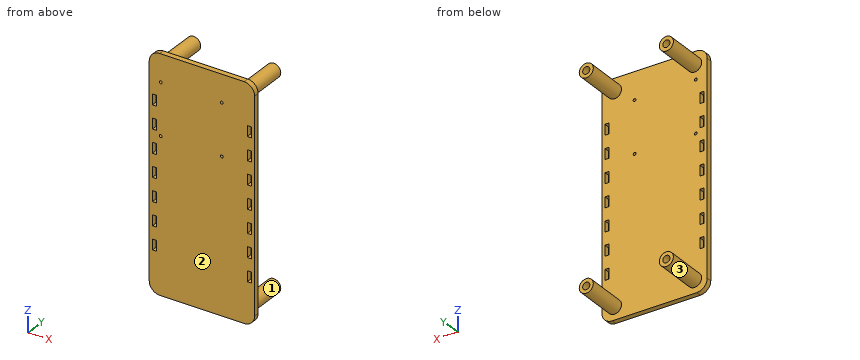
from build123d import *

# Parameters (mm, degrees)
SKETCH1_W           = 100
SKETCH1_H           = 220
BOSS_EXTRUDE1_DEPTH = 5
FILLET1_R           = 10
FILLET2_R           = 10
FILLET3_R           = 10
FILLET4_R           = 10
SKETCH2_R           = 6.668119003
BOSS_EXTRUDE2_DEPTH = 40
SKETCH4_R           = 3.418119003
CUT_EXTRUDE1_DEPTH  = 15
SKETCH5_R           = 3.418119003
CUT_EXTRUDE2_DEPTH  = 15
SKETCH6_R           = 3.418119003
CUT_EXTRUDE3_DEPTH  = 15
SKETCH7_R           = 3.418119003
CUT_EXTRUDE4_DEPTH  = 15
SKETCH8_W           = 4
SKETCH8_H           = 10
CUT_EXTRUDE5_DEPTH  = 157.908412776
SKETCH9_R           = 1.35
CUT_EXTRUDE7_DEPTH  = 159.256911381


with BuildPart() as part:
    # Sketch1 → Boss-Extrude1 (new body)
    with BuildSketch(Plane(origin=(0, 0, 0), x_dir=(1, 0, 0), z_dir=(0, 1, 0))):
        with Locations((-54.5, 0)):
            Rectangle(SKETCH1_W, SKETCH1_H)
    extrude(amount=BOSS_EXTRUDE1_DEPTH)

    # Fillet1
    fillet1_edges = [part.edges().sort_by_distance(p)[0] for p in [
        (-4.5, 2.5, 110),
    ]]
    fillet(fillet1_edges, radius=FILLET1_R)

    # Fillet2
    fillet2_edges = [part.edges().sort_by_distance(p)[0] for p in [
        (-4.5, 2.5, -110),
    ]]
    fillet(fillet2_edges, radius=FILLET2_R)

    # Fillet3
    fillet3_edges = [part.edges().sort_by_distance(p)[0] for p in [
        (-104.5, 2.5, 110),
    ]]
    fillet(fillet3_edges, radius=FILLET3_R)

    # Fillet4
    fillet4_edges = [part.edges().sort_by_distance(p)[0] for p in [
        (-104.5, 2.5, -110),
    ]]
    fillet(fillet4_edges, radius=FILLET4_R)

    # Sketch2 → Boss-Extrude2 (add)
    with BuildSketch(Plane(origin=(0, 5, 0), x_dir=(1, 0, 0), z_dir=(0, 1, 0))):
        with Locations(Location((-92.5, 98, 0), (0, 0, 270))):
            Circle(SKETCH2_R)
        with Locations(Location((-92.5, -98, 0), (0, 0, 90))):
            Circle(SKETCH2_R)
        with Locations(Location((-16.5, 98, 0), (0, 0, 90))):
            Circle(SKETCH2_R)
        with Locations(Location((-16.5, -98, 0), (0, 0, 270))):
            Circle(SKETCH2_R)
    extrude(amount=BOSS_EXTRUDE2_DEPTH)

    # Sketch4 → Cut-Extrude1 (cut)
    with BuildSketch(Plane(origin=(0, 45, 0), x_dir=(1, 0, 0), z_dir=(0, 1, 0))):
        with Locations(Location((-92.5, 98, 0), (0, 0, 270))):
            Circle(SKETCH4_R)
    extrude(amount=-CUT_EXTRUDE1_DEPTH, mode=Mode.SUBTRACT)

    # Sketch5 → Cut-Extrude2 (cut)
    with BuildSketch(Plane(origin=(0, 45, 0), x_dir=(1, 0, 0), z_dir=(0, 1, 0))):
        with Locations(Location((-92.5, -98, 0), (0, 0, 270))):
            Circle(SKETCH5_R)
    extrude(amount=-CUT_EXTRUDE2_DEPTH, mode=Mode.SUBTRACT)

    # Sketch6 → Cut-Extrude3 (cut)
    with BuildSketch(Plane(origin=(0, 45, 0), x_dir=(1, 0, 0), z_dir=(0, 1, 0))):
        with Locations(Location((-16.5, 98, 0), (0, 0, 270))):
            Circle(SKETCH6_R)
    extrude(amount=-CUT_EXTRUDE3_DEPTH, mode=Mode.SUBTRACT)

    # Sketch7 → Cut-Extrude4 (cut)
    with BuildSketch(Plane(origin=(0, 45, 0), x_dir=(1, 0, 0), z_dir=(0, 1, 0))):
        with Locations(Location((-16.5, -98, 0), (0, 0, 270))):
            Circle(SKETCH7_R)
    extrude(amount=-CUT_EXTRUDE4_DEPTH, mode=Mode.SUBTRACT)

    # Sketch8 → Cut-Extrude5 (cut, through all)
    with BuildSketch(Plane(origin=(0, 5, 0), x_dir=(1, 0, 0), z_dir=(0, 1, 0))):
        with Locations((-99.5, 66)):
            Rectangle(SKETCH8_W, SKETCH8_H)
        with Locations((-99.5, 44)):
            Rectangle(SKETCH8_W, SKETCH8_H)
        with Locations((-99.5, 22)):
            Rectangle(SKETCH8_W, SKETCH8_H)
        with Locations((-99.5, 0)):
            Rectangle(SKETCH8_W, SKETCH8_H)
        with Locations((-9.5, -66)):
            Rectangle(SKETCH8_W, SKETCH8_H)
        with Locations((-9.5, -44)):
            Rectangle(SKETCH8_W, SKETCH8_H)
        with Locations((-99.5, -22)):
            Rectangle(SKETCH8_W, SKETCH8_H)
        with Locations((-99.5, -44)):
            Rectangle(SKETCH8_W, SKETCH8_H)
        with Locations((-99.5, -66)):
            Rectangle(SKETCH8_W, SKETCH8_H)
        with Locations((-9.5, -22)):
            Rectangle(SKETCH8_W, SKETCH8_H)
        with Locations((-9.5, 0)):
            Rectangle(SKETCH8_W, SKETCH8_H)
        with Locations((-9.5, 22)):
            Rectangle(SKETCH8_W, SKETCH8_H)
        with Locations((-9.5, 44)):
            Rectangle(SKETCH8_W, SKETCH8_H)
        with Locations((-9.5, 66)):
            Rectangle(SKETCH8_W, SKETCH8_H)
    extrude(amount=-CUT_EXTRUDE5_DEPTH, mode=Mode.SUBTRACT)

    # Sketch9 → Cut-Extrude7 (cut, through all)
    with BuildSketch(Plane.XZ):
        with Locations(Location((-93.622758359, 35.073260268, 0), (0, 0, 270))):
            Circle(SKETCH9_R)
        with Locations(Location((-35.622758359, 35.073260268, 0), (0, 0, 270))):
            Circle(SKETCH9_R)
        with Locations(Location((-35.622758359, 84.073260268, 0), (0, 0, 270))):
            Circle(SKETCH9_R)
        with Locations(Location((-93.622758359, 84.073260268, 0), (0, 0, 270))):
            Circle(SKETCH9_R)
    extrude(amount=-CUT_EXTRUDE7_DEPTH, mode=Mode.SUBTRACT)


solid = part.part
Input: part model. Units: mm. Frame: model coordinates. Face numbers are marked on the shaded views. Give positions to 0.01 mm unless a question says otherwise; leave off trailing zeros. Order: outer loops, then holes, each group sorted by start corner. A loop starts at its lowest first (then second) coordinate and runs counter-clockwise, first axis right, second up. Notation, with made-up numbers: (79.25, 26.5) - (94.25, 26.5) arc R25 cw to (94.25, 42.5) - close; hole circle Ø8 at (30.25, 62.25). An arc over 180 degrees is marked (long way). Answer as a JSON object with one key per item and string values. Group by question number.
Q1. First-contact query: pin 1 Ø4.5 at (x, y) = (-99, 2) entering from -Z; pin 2 Ø3 at (x, y) = (-9.5, 2) entering from +Z. Flat tips, straight axial feed; report the tip coordinate or a pass-through.
Q2. Mould query, pull axis X, two halves, no side actions, for the marked faces 1, 2 and 3. Classes: pulls with the +X half, pulls with the -X half, needs draft (parallel to the pull), parting line crosses it, or undercut.
Q3. Line query: probe 1 along X at (y, z) = (37.25, -98); probe 2 along Y at (x, z) = (-93, -83.5); probe 3 along Z at (x, y) = (-18.5, 39). Output: solid intervals per line, ascending.
Q4. Cut plane D-D, the plane y = 8. Output: boundary loops of the cut face in (x, z), then the cut area to 3 significant figures.
Q5. Cut plane B-B, the plane z = -98. Output: boundary loops of the cut face in (x, y), then the cut area to 3 significant figures.
Q6. Cut plane A-A, the plane z = 24.5. Output: boundary loops of the cut face in (x, y).
Q7. Cut plane C-C, the plane x = -16.5. Output: boundary loops of the cut face in (y, z), then the cut area to 3 significant figures.
Results:
{
 "1": {"pin 1": "z = -109.74", "pin 2": "z = 109.37"},
 "2": {"face 1": "undercut", "face 2": "needs draft", "face 3": "undercut"},
 "3": {"probe 1": "-99.17 to -95.92, -89.08 to -85.83, -23.17 to -19.92, -13.08 to -9.83", "probe 2": "0 to 5", "probe 3": "-104.36 to -100.77, -95.23 to -91.64, 91.64 to 95.23, 100.77 to 104.36"},
 "4": {"outline": "circle Ø13.34 at (-92.5, -98); circle Ø13.34 at (-92.5, 98); circle Ø13.34 at (-16.5, -98); circle Ø13.34 at (-16.5, 98)", "area": "559 mm^2"},
 "5": {"outline": "(-104.5, 0) - (-4.5, 0) - (-4.5, 5) - (-9.83, 5) - (-9.83, 45) - (-13.08, 45) - (-13.08, 30) - (-19.92, 30) - (-19.92, 45) - (-23.17, 45) - (-23.17, 5) - (-85.83, 5) - (-85.83, 45) - (-89.08, 45) - (-89.08, 30) - (-95.92, 30) - (-95.92, 45) - (-99.17, 45) - (-99.17, 5) - (-104.5, 5) - close", "area": "1,360 mm^2"},
 "6": {"outline": "(-104.5, 0) - (-101.5, 0) - (-101.5, 5) - (-104.5, 5) - close; (-97.5, 0) - (-11.5, 0) - (-11.5, 5) - (-97.5, 5) - close; (-7.5, 0) - (-4.5, 0) - (-4.5, 5) - (-7.5, 5) - close"},
 "7": {"outline": "(0, -110) - (5, -110) - (5, -104.67) - (45, -104.67) - (45, -101.42) - (30, -101.42) - (30, -94.58) - (45, -94.58) - (45, -91.33) - (5, -91.33) - (5, 91.33) - (45, 91.33) - (45, 94.58) - (30, 94.58) - (30, 101.42) - (45, 101.42) - (45, 104.67) - (5, 104.67) - (5, 110) - (0, 110) - close", "area": "1,960 mm^2"}
}
